```python
from build123d import *

# Parameters (mm, degrees)
F0_W     = 43
F0_H     = 46
F1_DEPTH = 7
F2_R     = 3
F3_T     = -2
F4_R     = 3.25
F5_DEPTH = 2
F6_W     = 51.836722
F6_H     = 50.070026
F7_DEPTH = 3


with BuildPart() as f1:
    # F0 (on Top) → F1 (new body)
    with BuildSketch(Plane.XY):
        Rectangle(F0_W, F0_H)
    extrude(amount=F1_DEPTH)

    # F2
    f2_edges = [f1.edges().sort_by_distance(p)[0] for p in [
        (0, -23, 0),
        (21.5, 0, 0),
        (0, 23, 0),
        (-21.5, 0, 0),
        (21.5, 23, 3.5),
        (21.5, -23, 3.5),
        (-21.5, 23, 3.5),
        (-21.5, -23, 3.5),
    ]]
    fillet(f2_edges, radius=F2_R)

    # F3
    f3_openings = [f1.faces().sort_by_distance(p)[0] for p in [
        (0, 0, 7),
    ]]
    offset(amount=F3_T, openings=f3_openings)

    # F4 (on face) → F5 (cut, through all)
    with BuildSketch(Plane.XY.offset(2)):
        Circle(F4_R)
    extrude(amount=-F5_DEPTH, mode=Mode.SUBTRACT)

    # F6 (on face) → F7 (cut)
    with BuildSketch(Plane.XY.offset(7)):
        Rectangle(F6_W, F6_H)
        with BuildLine():
            ThreePointArc((18.5, 22), (19.914214, 21.414214), (20.5, 20))
            Line((20.5, 20), (20.5, -20))
            ThreePointArc((20.5, -20), (19.914214, -21.414214), (18.5, -22))
            Line((18.5, -22), (-18.5, -22))
            ThreePointArc((-18.5, -22), (-19.914214, -21.414214), (-20.5, -20))
            Line((-20.5, -20), (-20.5, 20))
            ThreePointArc((-20.5, 20), (-19.914214, 21.414214), (-18.5, 22))
            Line((-18.5, 22), (18.5, 22))
        make_face(mode=Mode.SUBTRACT)
    extrude(amount=-F7_DEPTH, mode=Mode.SUBTRACT)


solid = f1.part
```
Design review of the part built by this model. Coordinates are the model's own, in mm. A direction names the side the tool comes from. Round coordinates to 2 decimals unless told otherwise and drop trailing zeros. Write each loop counter-clockwise with the first axis right and the second up, starting at its lowest first coordinate (ties: lowest second). Pieces come first, ordered by that corner, then holes. Notation, with made-up numbers: (12.25, 74) -> (51.25, 74) arc R22 cw to (51.25, 84) -> close; hole circle Ø6 at (39.25, -11). An arc over 180 degrees is marked (long way). Write item = value, one per line. Start each with the question number.
1) Take a section at B-B, the plane x = 0. State the section outline as (y, z) points.
2) Take a section at D-D, the plane y = 9. State the section outline as (x, z) points, plus the area to 3 significant figures.
3) Wall thickness on probe 1 along X at (y, z) = (16, 4.75); probe 2 along X at (y, z) = (-1, 3.75); probe 3 along Z at (x, y) = (1.5, -7): over which ranges is each line inside the solid? List them lowest first. Write a range as from..to.
4) Take a section at A-A, the plane y = 0. State the section outline as (x, z) points.
5) Take a section at C-C, the plane x = -4.5. State the section outline as (y, z) points, plus the area to 3 significant figures.
6) Tool access review of faces 1 (the face through (0.26, 22.14, 0.9)), 2 (the face through (19.5, 0, 5)), 3 (the face through (-20.5, 0, 6)): name each direction out of +Z, -Z, +X, -X, +Y, -Y from which nothing blocks a thin tool from reaching the whole face with its end or side.
7) Clearance check with flat-ended pins moving along their axes: pin 1 (1.5 mm diameter, centred on y = -8, z = 5.5, fed in from -X); pin 2 (6 mm diameter, centred on x = -14.5, y = 0, fed in from +Z); pin 3 (1.2 mm diameter, centred on x = -3, z = 5, fed in from -Y). State where each tip first meets the part, or that it passes through.
8) Mouldability with a two-part tool opening along X and no side actions: class faces 4 (the face through (0, -21, 5)), 5 (the face through (0, 21, 5)), 6 (the face through (-19.93, 21.4, 5.52)), 7 (the face through (20.5, 0, 6)) as +X half, -X half, draft (parallel to the pull), parting line (faces both ways), or undercut.
Results list:
q1.outline = (-23, 3) arc R3 ccw to (-20, 0) -> (-3.25, 0) -> (-3.25, 2) -> (-20, 2) arc R1 cw to (-21, 3) -> (-21, 7) -> (-22, 7) -> (-22, 4) -> (-23, 4) -> close; (3.25, 0) -> (20, 0) arc R3 ccw to (23, 3) -> (23, 4) -> (22, 4) -> (22, 7) -> (21, 7) -> (21, 3) arc R1 cw to (20, 2) -> (3.25, 2) -> close
q2.outline = (-21.5, 3) arc R3 ccw to (-18.5, 0) -> (18.5, 0) arc R3 ccw to (21.5, 3) -> (21.5, 4) -> (20.5, 4) -> (20.5, 7) -> (19.5, 7) -> (19.5, 3) arc R1 cw to (18.5, 2) -> (-18.5, 2) arc R1 cw to (-19.5, 3) -> (-19.5, 7) -> (-20.5, 7) -> (-20.5, 4) -> (-21.5, 4) -> close
q2.area = 96.6 mm²
q3.probe_1 = -20.5..-19.5, 19.5..20.5
q3.probe_2 = -21.5..-19.5, 19.5..21.5
q3.probe_3 = 0..2
q4.outline = (-21.5, 3) arc R3 ccw to (-18.5, 0) -> (-3.25, 0) -> (-3.25, 2) -> (-18.5, 2) arc R1 cw to (-19.5, 3) -> (-19.5, 7) -> (-20.5, 7) -> (-20.5, 4) -> (-21.5, 4) -> close; (3.25, 0) -> (18.5, 0) arc R3 ccw to (21.5, 3) -> (21.5, 4) -> (20.5, 4) -> (20.5, 7) -> (19.5, 7) -> (19.5, 3) arc R1 cw to (18.5, 2) -> (3.25, 2) -> close
q5.outline = (-23, 3) arc R3 ccw to (-20, 0) -> (20, 0) arc R3 ccw to (23, 3) -> (23, 4) -> (22, 4) -> (22, 7) -> (21, 7) -> (21, 3) arc R1 cw to (20, 2) -> (-20, 2) arc R1 cw to (-21, 3) -> (-21, 7) -> (-22, 7) -> (-22, 4) -> (-23, 4) -> close
q5.area = 103 mm²
q6.face_1 = -Z, +X, -X, +Y
q6.face_2 = +Z
q6.face_3 = +Z, -X, +Y, -Y
q7.pin_1 = -20.5
q7.pin_2 = 2
q7.pin_3 = -22
q8.face_4 = undercut
q8.face_5 = undercut
q8.face_6 = -X half
q8.face_7 = +X half
